For this review, take the finished solid that the model builds, in its own axes (mm). A direction names the side the tool comes from. Coordinates: 2 decimals unless noted, no trailing zeros. Write each loop counter-clockwise with the first axis right and the second up, starting at its lowest first coordinate (ties: lowest second). Pieces come first, ordered by that corner, then holes. Notation, with made-up numbers: M -12.75,21.5 L 18.25,21.5 A19 ccw 18.25,36.5 Z; hole C 70.25,30.25 d5. An arc over 180 degrees is marked long. One line per question, with ' | ' between items.
from build123d import *

# Parameters (mm, degrees)
EXTRUDE_1_DEPTH     = 8
FILLET_1_R          = 1
CUT_EXTRUDE_START   = -10
CUT_EXTRUDE_1_DEPTH = 10
CUT_EXTRUDE_2_DEPTH = 16.370426149


with BuildPart() as part:
    # 草图1 → 凸台-拉伸1 (new body)
    with BuildSketch(Plane.XY):
        with BuildLine():
            Line((1.294095226, -4.829629131), (2.588190451, -9.659258263))
            ThreePointArc((2.588190451, -9.659258263), (0, 10), (-2.588190451, -9.659258263))
            Line((-2.588190451, -9.659258263), (-1.294095226, -4.829629131))
            ThreePointArc((-1.294095226, -4.829629131), (0, 5), (1.294095226, -4.829629131))
        make_face()
    extrude(amount=EXTRUDE_1_DEPTH)

    # 圆角1
    fillet_1_edges = [part.edges().sort_by_distance(p)[0] for p in [
        (-1.294095226, -4.829629131, 4),
        (1.294095226, -4.829629131, 4),
    ]]
    fillet(fillet_1_edges, radius=FILLET_1_R)

    # 草图2 → 切除-拉伸1 (cut)
    with BuildSketch(Plane.XY.offset(8).offset(CUT_EXTRUDE_START)):
        with BuildLine():
            Line((-8.5, 5.267826876), (-8.5, -5.267826876))
            ThreePointArc((-8.5, -5.267826876), (-10, 0), (-8.5, 5.267826876))
        make_face()
        with BuildLine():
            Line((8.5, 5.267826876), (8.5, -5.267826876))
            ThreePointArc((8.5, -5.267826876), (10, 0), (8.5, 5.267826876))
        make_face()
    extrude(amount=CUT_EXTRUDE_1_DEPTH, mode=Mode.SUBTRACT)

    # 草图3 → 切除-拉伸2 (cut, through all)
    with BuildSketch(Plane(origin=(0, 0, 0), x_dir=(-1, 0, 0), z_dir=(0, 0, -1))):
        with BuildLine():
            Line((0, 8), (-0.534023884, 4.971400053))
            ThreePointArc((-0.534023884, 4.971400053), (0, 5), (0.534023884, 4.971400053))
            Line((0.534023884, 4.971400053), (0, 8))
        make_face()
    extrude(amount=-CUT_EXTRUDE_2_DEPTH, mode=Mode.SUBTRACT)


solid = part.part
1. For line 1 along Y through (x, z) = (3, 5); line 2 along X through (y, z) = (-3.25, 0.5); line 3 along X through (y, z) = (-8.5, 7.75), list the stretches that pass through material, from the lowest coordinate up.
Computed values:
line 1: y = -9.54 to -4, 4 to 9.54 | line 2: x = -8.5 to -3.8, 3.8 to 8.5 | line 3: x = -5.27 to -2.28, 2.28 to 5.27
2. Take a section at A-A on y = -1.25. State the section outline as (x, z) points.
Computed values:
outline: M -8.5,0 L -4.84,0 L -4.84,8 L -8.5,8 Z; M 4.84,0 L 8.5,0 L 8.5,8 L 4.84,8 Z
3. Draft analysis for pull direction Y (two halves, no side actions). For faces 1 (the cylindrical face through (6, -8, 4)), 2 (the cylindrical face through (-4.95, 0.71, 3.94)), 3 (the flat face through (-2, 5, 0)), 4 (the cylindrical face through (4.92, 0.89, 3.94)), state which applies: pulls with the +Y half, pulls with the -Y half, needs draft (parallel to the pull), parting line crosses it, or undercut.
Computed values:
face 1: pulls with the -Y half | face 2: undercut | face 3: needs draft | face 4: undercut
4. Clearance check with flat-ended pins moving along their axes: P1, Ø2, axis at x = 4, z = 2, coming from the +Y side; P2, Ø3, axis at x = -5.5, z = 7, coming from the +Y side; P3, Ø4, axis at x = 3, z = 7, coming from the +Y side. State where each tip first meets the part, or that it passes through.
Computed values:
P1: stops at y = 9.54 | P2: stops at y = 9.17 | P3: stops at y = 9.95
5. Take a section at D-D on x = 7. State the section outline as (y, z) points.
Computed values:
outline: M -7.14,0 L 7.14,0 L 7.14,8 L -7.14,8 Z
6. Take a section at B-B on x = -4. State the section outline as (y, z) points, plus the area to 3 significant figures.
Computed values:
outline: M -9.17,0 L -3,0 L -3,8 L -9.17,8 Z; M 3,0 L 9.17,0 L 9.17,8 L 3,8 Z | area: 98.6 mm2
7. Machinability: for faces 5 (the cylindrical face through (-6, -8, 4)), 6 (the cylindrical face through (-1.588, -5.039, 4.056)), 7 (the flat face through (2.052, -7.659, 3.944)), which of the approach directions +Z, -Z, +X, -X, +Y, -Y give a long, thin tool a straight path to every point of the face, cutting with its end or side? Answer none if there is none.
Computed values:
face 5: +Z, -Z, -X, -Y | face 6: +Z, -Z | face 7: +Z, -Z, -Y
8. Take a section at C-C on z = 7.25. State the section outline as (x, y) points.
Computed values:
outline: M -8.5,-5.27 A10 ccw -2.59,-9.66 L -1.53,-5.71 A1 ccw -2.08,-4.55 A5 cw -0.53,4.97 L 0,8 L 0.53,4.97 A5 cw 2.08,-4.55 A1 ccw 1.53,-5.71 L 2.59,-9.66 A10 ccw 8.5,-5.27 L 8.5,5.27 A10 ccw -8.5,5.27 Z
